from build123d import *

# Parameters (mm, degrees)
SKETCH_1_W          = 54
SKETCH_1_H          = 39.8
SKETCH_1_W_2        = 46
SKETCH_1_H_2        = 32
EXTRUDE_1_DEPTH     = 143
SKETCH_3_W          = 54
SKETCH_3_H          = 39.8
EXTRUDE_2_DEPTH     = 3
SKETCH_4_W          = 8
SKETCH_4_H          = 8
SKETCH_4_R          = 1.6
EXTRUDE_3_DEPTH     = 39.8
FILLET_2_R          = 2
SKETCH_5_W          = 54
SKETCH_5_H          = 39.8
CUT_EXTRUDE_1_DEPTH = 3
FILLET_3_R          = 2


with BuildPart() as part:
    # 草图1 → 凸台-拉伸1 (new body)
    with BuildSketch(Plane.XY):
        Rectangle(SKETCH_1_W, SKETCH_1_H)
        Rectangle(SKETCH_1_W_2, SKETCH_1_H_2, mode=Mode.SUBTRACT)
    extrude(amount=EXTRUDE_1_DEPTH)

    # 草图3 → 凸台-拉伸2 (add)
    with BuildSketch(Plane(origin=(0, 0, 0), x_dir=(-1, 0, 0), z_dir=(0, 0, -1))):
        Rectangle(SKETCH_3_W, SKETCH_3_H)
    extrude(amount=EXTRUDE_2_DEPTH)

    # 草图4 → 凸台-拉伸3 (add)
    # profile 1 of 4: a face of its own
    with BuildSketch(Plane(origin=(0, 19.9, 0), x_dir=(1, 0, 0), z_dir=(0, 1, 0))):
        with Locations((-31, -121)):
            Rectangle(SKETCH_4_W, SKETCH_4_H)
        with Locations(Location((-31, -121, 0), (0, 0, 270))):
            Circle(SKETCH_4_R, mode=Mode.SUBTRACT)
    # profile 2 of 4: a face of its own
    with BuildSketch(Plane(origin=(0, 19.9, 0), x_dir=(1, 0, 0), z_dir=(0, 1, 0))):
        with Locations((31, -121)):
            Rectangle(SKETCH_4_W, SKETCH_4_H)
        with Locations(Location((31, -121, 0), (0, 0, 270))):
            Circle(SKETCH_4_R, mode=Mode.SUBTRACT)
    # profile 3 of 4: a face of its own
    with BuildSketch(Plane(origin=(0, 19.9, 0), x_dir=(1, 0, 0), z_dir=(0, 1, 0))):
        with Locations((31, -19)):
            Rectangle(SKETCH_4_W, SKETCH_4_H)
        with Locations(Location((31, -19, 0), (0, 0, 270))):
            Circle(SKETCH_4_R, mode=Mode.SUBTRACT)
    # profile 4 of 4: a face of its own
    with BuildSketch(Plane(origin=(0, 19.9, 0), x_dir=(1, 0, 0), z_dir=(0, 1, 0))):
        with Locations((-31, -19)):
            Rectangle(SKETCH_4_W, SKETCH_4_H)
        with Locations(Location((-31, -19, 0), (0, 0, 270))):
            Circle(SKETCH_4_R, mode=Mode.SUBTRACT)
    extrude(amount=-EXTRUDE_3_DEPTH)

    # 圆角2
    fillet_2_edges = [part.edges().sort_by_distance(p)[0] for p in [
        (23, -16, 71.5),
        (23, 16, 71.5),
        (-23, 16, 71.5),
        (-23, -16, 71.5),
    ]]
    fillet(fillet_2_edges, radius=FILLET_2_R)

    # 草图5 → 切除-拉伸1 (cut)
    with BuildSketch(Plane.XY.offset(143)):
        Rectangle(SKETCH_5_W, SKETCH_5_H)
    extrude(amount=-CUT_EXTRUDE_1_DEPTH, mode=Mode.SUBTRACT)

    # 圆角3
    fillet_3_edges = [part.edges().sort_by_distance(p)[0] for p in [
        (-27, 0, 140),
        (27, 0, 140),
        (27, 0, -3),
        (-27, 0, -3),
        (27, 0, 125),
        (27, 0, 117),
        (35, 0, 117),
        (35, 0, 125),
        (-27, 0, 117),
        (-27, 0, 125),
        (-35, 0, 125),
        (-35, 0, 117),
        (27, 0, 23),
        (27, 0, 15),
        (35, 0, 15),
        (35, 0, 23),
        (-35, 0, 15),
        (-27, 0, 15),
        (-27, 0, 23),
        (-35, 0, 23),
    ]]
    fillet(fillet_3_edges, radius=FILLET_3_R)


solid = part.part
The listing builds one solid part. Answer for the finished solid, in the listing's coordinates (mm). A direction names the side the tool comes from. Give positions to 0.01 mm unless a question says otherwise; leave off trailing zeros. Write each loop counter-clockwise with the first axis right and the second up, starting at its lowest first coordinate (ties: lowest second). Pieces come first, ordered by that corner, then holes. Notation, with made-up numbers: (-6.75, 69.5) - (30.25, 69.5) arc R25 ccw to (30.25, 90.5) - close; hole circle Ø9 at (18, -26.5). An arc over 180 degrees is marked (long way). Use a Markdown table: item, result.
1. Section D-D on x = -5 is taken. Write down the section's boundary in (y, z).
Values follow:
| item | result |
|---|---|
| outline | (-19.9, -3) - (19.9, -3) - (19.9, 140) - (16, 140) - (16, 0) - (-16, 0) - (-16, 140) - (-19.9, 140) - close |
2. Each of these flat-tipped pins is pushed along its axis until it touches: P1, Ø12, axis at y = -2.5, z = 131.5, coming from the +X side; P2, Ø2, axis at x = -31.5, y = 0.5, coming from the +Z side; P3, Ø3, axis at y = 12, z = 95, coming from the +X side. Where does it stop, or does it pass through?
Values follow:
| item | result |
|---|---|
| P1 | stops at x = 27.68 |
| P2 | stops at z = 125 |
| P3 | stops at x = 27 |
3. Find the intervals of material crossed by probe 1 along X at (y, z) = (9, 121); probe 2 along X at (y, z) = (6.5, 63); probe 3 along Y at (x, z) = (19, 81), in increasing order. Write a range as from..to.
Values follow:
| item | result |
|---|---|
| probe 1 | x = -35..-32.6, -29.4..-23, 23..29.4, 32.6..35 |
| probe 2 | x = -27..-23, 23..27 |
| probe 3 | y = -19.9..-16, 16..19.9 |
4. For a pull along Z with two mould halves and no side action, classify faces 1 (the flat face through (23, 0, 69)), 2 (the cylindrical face through (-30.519, 0.279, 122.526)), 3 (the flat face through (-31, 0, 15)) as released by +Z, released by -Z, zero draft, split by the parting line, or undercut.
Values follow:
| item | result |
|---|---|
| face 1 | zero draft |
| face 2 | undercut |
| face 3 | released by -Z |
5. Section B-B on x = 31 is taken. Write down the section's boundary in (y, z), plus the area to 3 significant figures.
Values follow:
| item | result |
|---|---|
| outline | (-19.9, 15) - (19.9, 15) - (19.9, 17.4) - (-19.9, 17.4) - close; (-19.9, 20.6) - (19.9, 20.6) - (19.9, 23) - (-19.9, 23) - close; (-19.9, 117) - (19.9, 117) - (19.9, 119.4) - (-19.9, 119.4) - close; (-19.9, 122.6) - (19.9, 122.6) - (19.9, 125) - (-19.9, 125) - close |
| area | 382 mm² |
6. A tool of negligible diameter and unlimited length cuts with its end or side. For faces 4 (the flat face through (0, 16, 69)), 5 (the flat face through (-27, 0, 6)), 6 (the flat face through (31, 0, 15)), 7 (the flat face through (-31, 0, 23)), from which of +Z, -Z, +X, -X, +Y, -Y can it reach the whole face along a straight path? Write none if from no direction.
Values follow:
| item | result |
|---|---|
| face 4 | +Z |
| face 5 | -Z, -X, +Y, -Y |
| face 6 | -Z, +X, +Y, -Y |
| face 7 | -X, +Y, -Y |
7. Section A-A on z = 19 is taken. Write down the section's boundary in (x, y), plus the area to 3 significant figures.
Values follow:
| item | result |
|---|---|
| outline | (-35, -19.9) - (-32.6, -19.9) - (-32.6, 19.9) - (-35, 19.9) - close; (-29.4, -19.9) - (29.4, -19.9) - (29.4, 19.9) - (-29.4, 19.9) - close; (32.6, -19.9) - (35, -19.9) - (35, 19.9) - (32.6, 19.9) - close; hole (-23, -14) arc R2 ccw to (-21, -16) - (21, -16) arc R2 ccw to (23, -14) - (23, 14) arc R2 ccw to (21, 16) - (-21, 16) arc R2 ccw to (-23, 14) - close |
| area | 1,060 mm² |
8. Section C-C on z = 52 is taken. Write down the section's boundary in (x, y), plus the area to 3 significant figures.
Values follow:
| item | result |
|---|---|
| outline | (-27, -19.9) - (27, -19.9) - (27, 19.9) - (-27, 19.9) - close; hole (-23, -14) arc R2 ccw to (-21, -16) - (21, -16) arc R2 ccw to (23, -14) - (23, 14) arc R2 ccw to (21, 16) - (-21, 16) arc R2 ccw to (-23, 14) - close |
| area | 681 mm² |
